Autodesk Inventor part; units mm, degrees
ref_plane "YZ Plane" through (0, 0, 0) normal (1, 0, 0) x (0, 1, 0)
ref_plane "XZ Plane" through (0, 0, 0) normal (0, 1, 0) x (-1, 0, 0)
ref_plane "XY Plane" through (0, 0, 0) normal (0, 0, 1) x (1, 0, 0)
sketch "Skizze1" plane through (0, 0, 0) normal (0, 0, 1) x (1, 0, 0)
  line L0 (-37.707, 0) -> (50.8634, 0) construction
  line L1 (0, -35.4687) -> (0, 37.4335) construction
  line L2 (0, 0) -> (27.0189, 27.0189) construction
  line L3 (0, 0) -> (38.2105, 0) construction
  line L4 (0, 24.9041) -> (16.9, 24.9041)
  line L5 (16.9, 24.9041) -> (16.9, 21.2841)
  line L6 (16.9, 21.2841) -> (19.092, 19.092)
  line L7 (24.9041, 0) -> (24.9041, 16.9)
  line L8 (24.9041, 16.9) -> (21.2841, 16.9)
  line L9 (21.2841, 16.9) -> (19.092, 19.092)
  line L10 (0, 24.9041) -> (-16.9, 24.9041)
  line L11 (-16.9, 24.9041) -> (-16.9, 21.2841)
  line L12 (-16.9, 21.2841) -> (-19.092, 19.092)
  line L13 (-24.9041, 0) -> (-24.9041, 16.9)
  line L14 (-24.9041, 16.9) -> (-21.2841, 16.9)
  line L15 (-21.2841, 16.9) -> (-19.092, 19.092)
  line L16 (0, -24.9041) -> (16.9, -24.9041)
  line L17 (16.9, -24.9041) -> (16.9, -21.2841)
  line L18 (16.9, -21.2841) -> (19.092, -19.092)
  line L19 (24.9041, 0) -> (24.9041, -16.9)
  line L20 (24.9041, -16.9) -> (21.2841, -16.9)
  line L21 (21.2841, -16.9) -> (19.092, -19.092)
  line L22 (0, -24.9041) -> (-16.9, -24.9041)
  line L23 (-16.9, -24.9041) -> (-16.9, -21.2841)
  line L24 (-16.9, -21.2841) -> (-19.092, -19.092)
  line L25 (-24.9041, 0) -> (-24.9041, -16.9)
  line L26 (-24.9041, -16.9) -> (-21.2841, -16.9)
  line L27 (-21.2841, -16.9) -> (-19.092, -19.092)
  circle A0 centre (0, 0) radius 18
  circle A1 centre (-16.6172, 16.6172) radius 1.5
  line L28 (-16.6172, 16.6172) -> (16.6172, 16.6172) construction
  line L29 (16.6172, 16.6172) -> (16.6172, -16.6172) construction
  line L30 (16.6172, -16.6172) -> (-16.6172, -16.6172) construction
  line L31 (-16.6172, -16.6172) -> (-16.6172, 16.6172) construction
  circle A2 centre (16.6172, 16.6172) radius 1.5
  circle A3 centre (-16.6172, -16.6172) radius 1.5
  circle A4 centre (16.6172, -16.6172) radius 1.5
  line L32 (-17.05, 25.0541) -> (0, 25.0541)
  line L33 (0, 25.0541) -> (17.05, 25.0541)
  line L34 (17.05, 25.0541) -> (17.05, 21.3462)
  line L35 (17.05, 21.3462) -> (19.1981, 19.1981)
  line L36 (19.1981, 19.1981) -> (21.3462, 17.05)
  line L37 (21.3462, 17.05) -> (25.0541, 17.05)
  line L38 (25.0541, 17.05) -> (25.0541, 0)
  line L39 (25.0541, 0) -> (25.0541, -17.05)
  line L40 (25.0541, -17.05) -> (21.3462, -17.05)
  line L41 (21.3462, -17.05) -> (19.1981, -19.1981)
  line L42 (19.1981, -19.1981) -> (17.05, -21.3462)
  line L43 (17.05, -21.3462) -> (17.05, -25.0541)
  line L44 (17.05, -25.0541) -> (0, -25.0541)
  line L45 (0, -25.0541) -> (-17.05, -25.0541)
  line L46 (-17.05, -25.0541) -> (-17.05, -21.3462)
  line L47 (-17.05, -21.3462) -> (-19.1981, -19.1981)
  line L48 (-19.1981, -19.1981) -> (-21.3462, -17.05)
  line L49 (-21.3462, -17.05) -> (-25.0541, -17.05)
  line L50 (-25.0541, -17.05) -> (-25.0541, 0)
  line L51 (-25.0541, 0) -> (-25.0541, 17.05)
  line L52 (-25.0541, 17.05) -> (-21.3462, 17.05)
  line L53 (-21.3462, 17.05) -> (-19.1981, 19.1981)
  line L54 (-19.1981, 19.1981) -> (-17.05, 21.3462)
  line L55 (-17.05, 21.3462) -> (-17.05, 25.0541)
  dimension "d0" = 45
  dimension "d1" = 16.9
  dimension "d2" = 3.62
  dimension "d3" = 3.1
  dimension "d4" = 36
  dimension "d7" = 3
  dimension "d8" = 3
  dimension "d9" = 3
  dimension "d10" = 3
  dimension "d11" = 3.5
  dimension "d12" = 0.15
extrude "Extrusion1" add sketch "Skizze1" along normal blind 2.5 contours L4 L5 L6 L9 L8 L7 L19 L20 L21 L18 L17 L16 L22 L23 L24 L27 L26 L25 L13 L14 L15 L12 L11 L10 | L32 L33 L34 L35 L36 L37 L38 L39 L40 L41 L42 L43 L44 L45 L46 L47 L48 L49 L50 L51 L52 L53 L54 L55
equation "\"d8\" = d7"
equation "\"d9\" = d7"
equation "\"d10\" = d7"
properties part number "LC_lens_holder_outer"
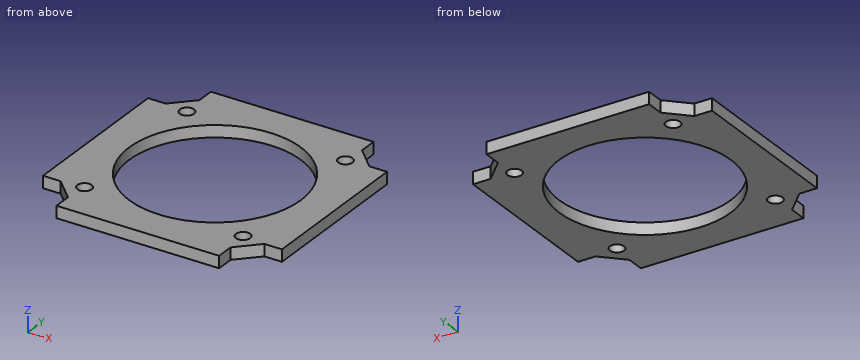
Build history of the part. All positions in model axes, mm. Give positions to 0.01 mm unless a question says otherwise; leave off trailing zeros. Loops run counter-clockwise (first coordinate to the right, second up) from the corner with the lowest first, then second, coordinate; pieces in that order, holes last.
Item 1: Slice it at D-D, the plane y = -16. List the corners of the cut face in (x, z).
Answers follow:
outline: (-25.05, 0) - (-17.98, 0) - (-17.98, 2.5) - (-25.05, 2.5) - close; (-15.25, 0) - (-8.25, 0) - (-8.25, 2.5) - (-15.25, 2.5) - close; (8.25, 0) - (15.25, 0) - (15.25, 2.5) - (8.25, 2.5) - close; (17.98, 0) - (25.05, 0) - (25.05, 2.5) - (17.98, 2.5) - close
Item 2: Slice it at A-A, the plane y = 0. List the corners of the cut face in (x, z).
Answers follow:
outline: (-25.05, 0) - (-18, 0) - (-18, 2.5) - (-25.05, 2.5) - close; (18, 0) - (25.05, 0) - (25.05, 2.5) - (18, 2.5) - close
Item 3: Drill centre lines: line 1 (Y direction, x = 0, z = 1.3); line 2 (Y direction, x = -16.5, z = 0.5); line 3 (Y direction, x = -15, z = 0.5). Where is each one in solid material? Low to high.
Answers follow:
line 1: y = -25.05 to -18, 18 to 25.05
line 2: y = -25.05 to -18.11, -15.12 to -7.19, 7.19 to 15.12, 18.11 to 25.05
line 3: y = -25.05 to -9.95, 9.95 to 25.05
Item 4: Slice it at C-C, the plane z = 1.55. List the corners of the cut face in (x, y), and give its area (3 significant figures).
Answers follow:
outline: (-25.05, -17.05) - (-21.35, -17.05) - (-17.05, -21.35) - (-17.05, -25.05) - (17.05, -25.05) - (17.05, -21.35) - (21.35, -17.05) - (25.05, -17.05) - (25.05, 17.05) - (21.35, 17.05) - (17.05, 21.35) - (17.05, 25.05) - (-17.05, 25.05) - (-17.05, 21.35) - (-21.35, 17.05) - (-25.05, 17.05) - close; hole circle Ø3 at (-16.62, -16.62); hole circle Ø3 at (-16.62, 16.62); hole circle Ø36 at (0, 0); hole circle Ø3 at (16.62, -16.62); hole circle Ø3 at (16.62, 16.62)
area: 1,250 mm2
Item 5: Flat gauge pins, fed straight in: pin 1 (1.2 mm diameter, centred on y = 23, z = 1, fed in from -X); pin 2 (2.5 mm diameter, centred on x = 16.62, y = 16.62, fed in from -Z). Where does each tip first touch, or does it go through?
Answers follow:
pin 1: stops at x = -17.05
pin 2: passes through
